from build123d import *

# Parameters (mm, degrees)
F0_W     = 7.25
F0_H     = 4.7
F0_W_2   = 6.25
F0_H_2   = 3.7
F1_DEPTH = 2.8
F0_W_3   = 4
F0_H_3   = 2
F2_DEPTH = 0.65
F3_R     = 0.5
F5_DEPTH = 25
F6_R     = 0.2


with BuildPart() as f1:
    # F0 (on Top) → F1 (new body)
    with BuildSketch(Plane.XY):
        with Locations((-7.525, -4.5)):
            Rectangle(F0_W, F0_H)
        with Locations((-7.525, -4.5)):
            Rectangle(F0_W_2, F0_H_2, mode=Mode.SUBTRACT)
    extrude(amount=F1_DEPTH)

    # F0 (on Top) → F2 (join)
    with BuildSketch(Plane.XY):
        with Locations((-7.525, -4.5)):
            Rectangle(F0_W_2, F0_H_2)
        with Locations((-7.525, -4.5)):
            Rectangle(F0_W_3, F0_H_3, mode=Mode.SUBTRACT)
    extrude(amount=F2_DEPTH)

    # F3
    f3_edges = [f1.edges().sort_by_distance(p)[0] for p in [
        (-7.525, -2.15, 0),
        (-11.15, -4.5, 0),
        (-7.525, -6.85, 0),
        (-3.9, -4.5, 0),
        (-5.525, -4.5, 0),
        (-7.525, -5.5, 0),
        (-9.525, -4.5, 0),
        (-7.525, -3.5, 0),
    ]]
    fillet(f3_edges, radius=F3_R)

    # F4 (on face) → F5 (cut)
    with BuildSketch(Plane.YZ.offset(-3.9)):
        with BuildLine():
            ThreePointArc((-5.65, 2.8), (-4.5, 1.65), (-3.35, 2.8))
            Line((-3.35, 2.8), (-5.65, 2.8))
        make_face()
    extrude(amount=-F5_DEPTH, mode=Mode.SUBTRACT)

    # F6
    f6_edges = [f1.edges().sort_by_distance(p)[0] for p in [
        (-7.525, -2.65, 0.65),
        (-10.65, -4.5, 0.65),
        (-7.525, -6.35, 0.65),
        (-4.4, -4.5, 0.65),
        (-9.525, -4.5, 0.65),
        (-7.525, -3.5, 0.65),
        (-5.525, -4.5, 0.65),
        (-7.525, -5.5, 0.65),
        (-10.65, -4.5, 1.65),
        (-4.4, -4.5, 1.65),
        (-10.65, -3, 2.8),
        (-3.9, -2.15, 1.65),
        (-3.9, -6.85, 1.65),
        (-11.15, -2.15, 1.65),
        (-11.15, -6.85, 1.65),
        (-4.4, -3, 2.8),
        (-4.4, -6, 2.8),
        (-10.65, -6, 2.8),
    ]]
    fillet(f6_edges, radius=F6_R)


solid = f1.part
Build history of the part. All positions in model axes, mm. A direction names the side the tool comes from. Round coordinates to 2 decimals unless told otherwise and drop trailing zeros. Write each loop counter-clockwise with the first axis right and the second up, starting at its lowest first coordinate (ties: lowest second). Pieces come first, ordered by that corner, then holes. Notation, with made-up numbers: M 8.25,20 L 45.25,20 A19 cw 45.25,47 Z; hole C 10,-16 d11. An arc over 180 degrees is marked long. Use CSV: the item, a comma, the result in double quotes.
1. Flat gauge pins, fed straight in: pin 1 (1.7 mm diameter, centred on x = -8.5, y = -5, fed in from +Z); pin 2 (1.4 mm diameter, centred on y = -4.5, z = 2, fed in from -X). Where does each tip first touch, or does it go through?
Reply:
pin 1,"stops at z = 0.65"
pin 2,"stops at x = -11.15"
2. Two-plate mould, pull along Y, no slides. Class faces 1 (the face through (-7.6, -6.6, 2.8)), 2 (the face through (-8, -2.15, 2)), 3 (the face through (-4.4, -5, 1)): +Y half, -Y half, draft (parallel to the pull), parting line (faces both ways), or undercut.
Reply:
face 1,"draft"
face 2,"+Y half"
face 3,"undercut"
3. Wall check: probe 1 along Y at (x, z) = (-6.75, 1.5); probe 2 along X at (y, z) = (-6.1, 1.75); probe 3 along Y at (x, z) = (-6.5, 0.2). Give the ranges that are in metal, low to high. Write a range as from..to.
Reply:
probe 1,"y = -6.85..-6.35, -2.65..-2.15"
probe 2,"x = -11.15..-10.65, -4.4..-3.9"
probe 3,"y = -6.75..-5.6, -3.4..-2.25"
4. Saw through at A-A (z = 1.1). Give the cut face in (x, y).
Reply:
outline,"M -11.15,-6.65 A0.2 ccw -10.95,-6.85 L -4.1,-6.85 A0.2 ccw -3.9,-6.65 L -3.9,-2.35 A0.2 ccw -4.1,-2.15 L -10.95,-2.15 A0.2 ccw -11.15,-2.35 Z; hole M -10.65,-6.35 L -4.4,-6.35 L -4.4,-2.65 L -10.65,-2.65 Z"
5. Tool access for faces 4 (the face through (-3.9, -5, 1)), 5 (the face through (-10.65, -5, 1)): list every direction of +Z, -Z, +X, -X, +Y, -Y with a clear straight run to the whole face (end or side of a thin tool).
Reply:
face 4,"+Z, -Z, +X, +Y, -Y"
face 5,"+Z"
